Check sheet for the modelled part. Datum: model origin and axes. Units: mm. A direction names the side the tool comes from. Round coordinates to 2 decimals unless told otherwise and drop trailing zeros. Write each loop counter-clockwise with the first axis right and the second up, starting at its lowest first coordinate (ties: lowest second). Pieces come first, ordered by that corner, then holes. Notation, with made-up numbers: (17.25, -11.75) -> (51.25, -11.75) arc R20 cw to (51.25, 10.25) -> close; hole circle Ø2 at (-24.75, 36). An arc over 180 degrees is marked (long way). One line per item, written item: value.
from build123d import *

# Parameters (mm, degrees)
SKETCH1_R           = 9.99
BOSS_EXTRUDE1_DEPTH = 16
SKETCH3_R           = 17.5
BOSS_EXTRUDE2_DEPTH = 1.8
SKETCH4_R           = 4.5
CUT_EXTRUDE1_DEPTH  = 16
SKETCH6_R           = 1.75
CUT_EXTRUDE2_DEPTH  = 1.8
CIRPATTERN1_COUNT   = 6


with BuildPart() as part:
    # Sketch1 → Boss-Extrude1 (new body)
    with BuildSketch(Plane(origin=(0, 0, 0), x_dir=(1, 0, 0), z_dir=(0, 1, 0))):
        with Locations(Location((0, 0, 0), (0, 0, 270))):
            Circle(SKETCH1_R)
    extrude(amount=BOSS_EXTRUDE1_DEPTH)

    # Sketch3 → Boss-Extrude2 (add)
    with BuildSketch(Plane.XZ):
        with Locations(Location((0, 0, 0), (0, 0, 270))):
            Circle(SKETCH3_R)
    extrude(amount=-BOSS_EXTRUDE2_DEPTH)

    # Sketch4 → Cut-Extrude1 (cut)
    with BuildSketch(Plane.XZ):
        with Locations(Location((0, 0, 0), (0, 0, 270))):
            Circle(SKETCH4_R)
    extrude(amount=-CUT_EXTRUDE1_DEPTH, mode=Mode.SUBTRACT)

    # Sketch6 → Cut-Extrude2 (cut)
    with BuildSketch(Plane.XZ):
        with Locations(Location((13.5, 0, 0), (0, 0, 270))):
            Circle(SKETCH6_R)
    cut_extrude2 = extrude(amount=-CUT_EXTRUDE2_DEPTH, mode=Mode.SUBTRACT)

    # CirPattern1: Cut-Extrude2 ×6 about axis
    cirpattern1_axis = Axis((0, 0, 0), (0, 1, 0))
    for i in range(1, CIRPATTERN1_COUNT):
        add(cut_extrude2.rotate(cirpattern1_axis, i * 360 / CIRPATTERN1_COUNT), mode=Mode.SUBTRACT)


solid = part.part
Item 1: Sectioned sample at A-A on x = 0. Enter the section's corners in (y, z).
Answer:
outline: (0, -17.5) -> (1.8, -17.5) -> (1.8, -9.99) -> (16, -9.99) -> (16, -4.5) -> (0, -4.5) -> close; (0, 4.5) -> (16, 4.5) -> (16, 9.99) -> (1.8, 9.99) -> (1.8, 17.5) -> (0, 17.5) -> close
Item 2: Thickness scan on line 1 (X direction, y = 6.75, z = 0); line 2 (Y direction, x = 7, z = 16); line 3 (X direction, y = 6.5, z = 1.5). Record the ranges inside material, lowest first.
Answer:
line 1: x = -9.99 to -4.5, 4.5 to 9.99
line 2: y = 0 to 1.8
line 3: x = -9.88 to -4.24, 4.24 to 9.88
Item 3: Depth check by flat-ended pin: P1, Ø5.5, axis at x = 13.5, z = 0, coming from the +Y side; P2, Ø3, axis at y = 11, z = -2, coming from the -X side; P3, Ø3, axis at y = 10.5, z = 9.5, coming from the +X side. Enter the tip coordinate at first touch or a pass-through.
Answer:
P1: stops at y = 1.8
P2: stops at x = -9.98
P3: stops at x = 5.98
Item 4: Sectioned sample at C-C on x = 6.75. Enter the section's corners in (y, z), and give its area (3 significant figures).
Answer:
outline: (0, -16.15) -> (1.8, -16.15) -> (1.8, -13.44) -> (0, -13.44) -> close; (0, -9.94) -> (1.8, -9.94) -> (1.8, -7.36) -> (16, -7.36) -> (16, 7.36) -> (1.8, 7.36) -> (1.8, 9.94) -> (0, 9.94) -> close; (0, 13.44) -> (1.8, 13.44) -> (1.8, 16.15) -> (0, 16.15) -> close
area: 255 mm^2
Item 5: Sectioned sample at D-D on y = 9.5. Enter the section's corners in (x, z).
Answer:
outline: circle Ø19.98 at (0, 0); hole circle Ø9 at (0, 0)
Item 6: Mould release check, pull along Z, two halves, no side actions. Record for faces 3 (the cylindrical face through (15.235, 0.887, 0.228)), 4 (the flat face through (-2.1, 16, 4.3)), 5 (the cylindrical face through (-10.648, 0.887, 13.887)): pulls with the +Z half, pulls with the -Z half, needs draft (parallel to the pull), parting line crosses it, or undercut.
Answer:
face 3: undercut
face 4: needs draft
face 5: parting line crosses it
Item 7: Tool access check on faces 1 (the cylindrical face through (8.424, 8.801, 5.371)), 2 (the cylindrical face through (-7.42, 0.89, -13.31)). Record the directions out of +Z, -Z, +X, -X, +Y, -Y that give a thin tool (end or side, any length) a straight path to the whole face; none if there is none.
Answer:
face 1: +Y
face 2: +Y, -Y
Item 8: Sectioned sample at B-B on z = 0. Enter the section's corners in (x, y).
Answer:
outline: (-17.5, 0) -> (-15.25, 0) -> (-15.25, 1.8) -> (-17.5, 1.8) -> close; (-11.75, 0) -> (-4.5, 0) -> (-4.5, 16) -> (-9.99, 16) -> (-9.99, 1.8) -> (-11.75, 1.8) -> close; (4.5, 0) -> (11.75, 0) -> (11.75, 1.8) -> (9.99, 1.8) -> (9.99, 16) -> (4.5, 16) -> close; (15.25, 0) -> (17.5, 0) -> (17.5, 1.8) -> (15.25, 1.8) -> close
